Could you check a few things on this model? Use its own coordinates, in mm. Give positions to 0.01 mm unless a question says otherwise; leave off trailing zeros. Order: outer loops, then holes, each group sorted by start corner. A loop starts at its lowest first (then second) coordinate and runs counter-clockwise, first axis right, second up. Notation, with made-up numbers: (30, -27.75) - (46, -27.75) arc R15 ccw to (46, -0.75) - close; hole circle Ø1 at (1, 80). An arc over 180 degrees is marked (long way). One line per question, with ' | ' between items. Start each with the question number.
1. For P1, Ø3.5, axis at x = -179.705, z = 86.36, coming from the +Y side; P2, Ø1.8, axis at y = 1, z = 1.5, coming from the -X side; P3, Ø0.5, axis at x = -257.5, y = 1.5, coming from the +Z side, each with a flat end and sliding along its axis, tell me the tip position at first contact or that it passes through.
2. Imagine slicing it at A-A (x = -237.5). Please give me the cut outline in (y, z) (3 decimals).
3. I need wall thicknesses on probe 1 along Z at (x, y) = (-246.38, 1.7); probe 2 along X at (y, z) = (1.45, 378.46); probe 3 along X at (y, z) = (1.5, 127). Which ranges of each line are inside material? Lowest first, please. Write a range as from..to.
```python
from build123d import *

# Parameters (mm, degrees)
SKETCH1_W             = 259.08
SKETCH1_H             = 391.16
BOSS_EXTRUDE1_DEPTH   = 3.175
F_8_CLEARANCE_HOLE1_D = 4.4958
F_8_CLEARANCE_HOLE2_D = 4.4958
SKETCH25_W            = 3.81
SKETCH25_H            = 24.13
SKETCH25_H_2          = 3.81
SKETCH25_W_2          = 24.13
CUT_EXTRUDE1_DEPTH    = 470.18937821
FILLET2_R             = 1.5875
FILLET3_R             = 6.35
MIRROR1_DEPTH         = 3.175


# Read off the part's stored shape, not the designer's step: Mirror1
with BuildPart() as part:
    # Sketch1 → Boss-Extrude1 (new body)
    with BuildSketch(Plane(origin=(0, 0, 0), x_dir=(1, 0, 0), z_dir=(0, 1, 0))):
        with Locations((-129.54, -195.58)):
            Rectangle(SKETCH1_W, SKETCH1_H)
    extrude(amount=BOSS_EXTRUDE1_DEPTH)

    # #8 Clearance Hole1 (through all)
    with Locations(Plane(origin=(0, 0, 0), x_dir=(-1, 0, 0), z_dir=(0, -1, 0))):
        with Locations((84.455, -63.5), (84.455, -86.36), (179.705, -86.36), (179.705, -63.5)):
            Hole(F_8_CLEARANCE_HOLE1_D / 2)

    # #8 Clearance Hole2 (through all)
    with Locations(Plane(origin=(0, 0, 0), x_dir=(-1, 0, 0), z_dir=(0, -1, 0))):
        with Locations((12.7, -101.6), (220.98, -12.7), (246.38, -101.6), (246.38, -289.56), (195.58, -12.7), (12.7, -289.56), (246.38, -264.16), (246.38, -127), (12.7, -127), (12.7, -264.16), (12.7, -378.46), (220.98, -378.46), (38.1, -12.7), (12.7, -12.7), (38.1, -378.46), (195.58, -378.46)):
            Hole(F_8_CLEARANCE_HOLE2_D / 2)

    # Sketch25 → Cut-Extrude1 (cut, through all)
    with BuildSketch(Plane.XZ):
        with Locations((-257.175, 375.285)):
            Rectangle(SKETCH25_W, SKETCH25_H)
        with Locations((-257.175, 389.255)):
            Rectangle(SKETCH25_W, SKETCH25_H_2)
        with Locations((-243.205, 389.255)):
            Rectangle(SKETCH25_W_2, SKETCH25_H_2)
    extrude(amount=-CUT_EXTRUDE1_DEPTH, mode=Mode.SUBTRACT)

    # Fillet2
    fillet2_edges = [part.edges().sort_by_distance(p)[0] for p in [
        (-255.27, 1.5875, 363.22),
        (-259.08, 1.5875, 363.22),
        (-231.14, 1.5875, 391.16),
        (-231.14, 1.5875, 387.35),
    ]]
    fillet(fillet2_edges, radius=FILLET2_R)

    # Fillet3
    fillet3_edges = [part.edges().sort_by_distance(p)[0] for p in [
        (-255.27, 1.5875, 387.35),
    ]]
    fillet(fillet3_edges, radius=FILLET3_R)

    # Mirror1 outline → Mirror1 (cut)
    with BuildSketch(Plane(origin=(0, 0, 0), x_dir=(1, 0, 0), z_dir=(0, 1, 0))):
        with BuildLine():
            ThreePointArc((-256.8575, -27.94), (-255.734967985, -27.475032015), (-255.27, -26.3525))
            Line((-255.27, -26.3525), (-255.27, -10.16))
            ThreePointArc((-255.27, -10.16), (-253.410128061, -5.669871939), (-248.92, -3.81))
            Line((-248.92, -3.81), (-232.7275, -3.81))
            ThreePointArc((-232.7275, -3.81), (-231.604967985, -3.345032015), (-231.14, -2.2225))
            Line((-231.14, -2.2225), (-231.14, 0))
            Line((-231.14, 0), (-259.08, 0))
            Line((-259.08, 0), (-259.08, -29.5275))
            ThreePointArc((-259.08, -29.5275), (-258.615032015, -28.404967985), (-257.4925, -27.94))
            Line((-257.4925, -27.94), (-256.8575, -27.94))
        make_face()
    extrude(amount=MIRROR1_DEPTH, mode=Mode.SUBTRACT)


solid = part.part
```
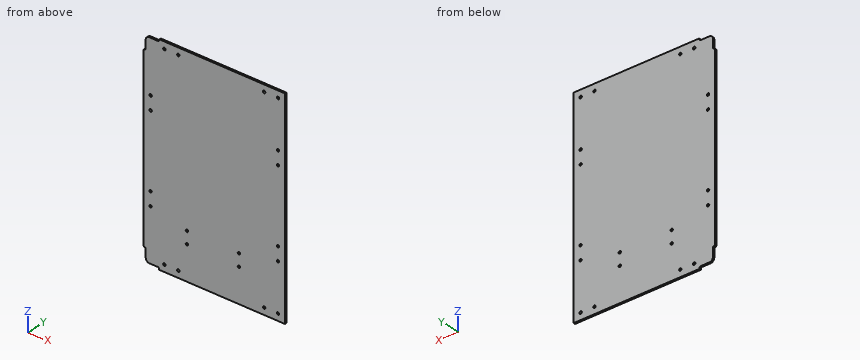
Results found:
1) P1: passes through | P2: stops at x = -231.15 | P3: stops at z = 363.22
2) outline: (0, 3.81) - (3.175, 3.81) - (3.175, 387.35) - (0, 387.35) - close
3) probe 1: z = 3.81..99.35, 103.85..124.75, 129.25..261.91, 266.41..287.31, 291.81..387.35 | probe 2: x = -255.27..-223.23, -218.73..-197.83, -193.33..-40.35, -35.85..-14.95, -10.45..0 | probe 3: x = -259.08..-248.63, -244.13..-14.95, -10.45..0
